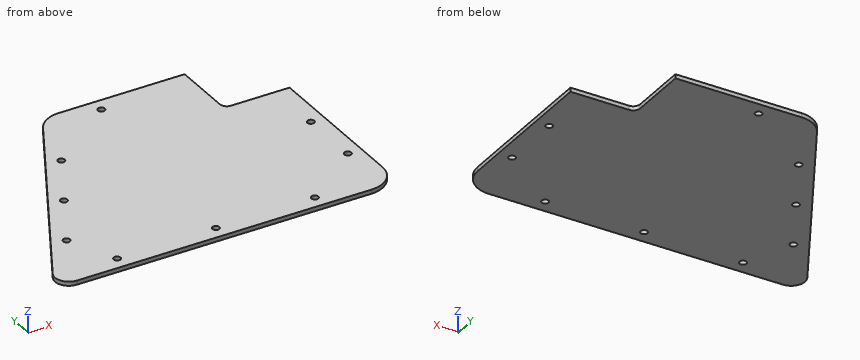
```python
from build123d import *

# Parameters (mm, degrees)
BOSS_EXTRUDE1_DEPTH = 3
CUT_EXTRUDE1_REACH  = 245.11
SKETCH2_R           = 2.5
CUT_EXTRUDE2_DEPTH  = 244.110466883


with BuildPart() as part:
    # Sketch1 → Boss-Extrude1 (new body)
    with BuildSketch(Plane.XY):
        with BuildLine():
            Line((-59.436088262, 179.5), (59.436088262, 179.5))
            ThreePointArc((59.436088262, 179.5), (73.578223886, 173.642135624), (79.436088262, 159.5))
            Line((79.436088262, 159.5), (79.436088262, 20))
            ThreePointArc((79.436088262, 20), (73.578223886, 5.857864376), (59.436088262, 0))
            Line((59.436088262, 0), (-153.931232863, 0))
            ThreePointArc((-153.931232863, 0), (-162.549941964, 4.928722701), (-162.672805625, 14.856429312))
            Line((-162.672805625, 14.856429312), (-76.919233785, 169.212858624))
            ThreePointArc((-76.919233785, 169.212858624), (-69.57864286, 176.737418201), (-59.436088262, 179.5))
        make_face()
    extrude(amount=BOSS_EXTRUDE1_DEPTH)

    # Sketch2 → Cut-Extrude1 (cut, up to next)
    with BuildSketch(Plane.XY.offset(3), mode=Mode.PRIVATE) as cut_extrude1_sk1:
        with Locations((-34.436088262, 169.5)):
            Circle(SKETCH2_R)
    cut_extrude1_tool1 = extrude(cut_extrude1_sk1.sketch, amount=-CUT_EXTRUDE1_REACH, mode=Mode.PRIVATE) & part.part
    # Sketch2 → Cut-Extrude1 (cut, up to next)
    with BuildSketch(Plane.XY.offset(3), mode=Mode.PRIVATE) as cut_extrude1_sk2:
        with Locations((34.433911738, 169.5)):
            Circle(SKETCH2_R)
    cut_extrude1_tool2 = extrude(cut_extrude1_sk2.sketch, amount=-CUT_EXTRUDE1_REACH, mode=Mode.PRIVATE) & part.part
    # Sketch2 → Cut-Extrude1 (cut, up to next)
    with BuildSketch(Plane.XY.offset(3), mode=Mode.PRIVATE) as cut_extrude1_sk3:
        with Locations((69.436088262, 134.5)):
            Circle(SKETCH2_R)
    cut_extrude1_tool3 = extrude(cut_extrude1_sk3.sketch, amount=-CUT_EXTRUDE1_REACH, mode=Mode.PRIVATE) & part.part
    # Sketch2 → Cut-Extrude1 (cut, up to next)
    with BuildSketch(Plane.XY.offset(3), mode=Mode.PRIVATE) as cut_extrude1_sk4:
        with Locations((69.436088262, 89.75)):
            Circle(SKETCH2_R)
    cut_extrude1_tool4 = extrude(cut_extrude1_sk4.sketch, amount=-CUT_EXTRUDE1_REACH, mode=Mode.PRIVATE) & part.part
    # Sketch2 → Cut-Extrude1 (cut, up to next)
    with BuildSketch(Plane.XY.offset(3), mode=Mode.PRIVATE) as cut_extrude1_sk5:
        with Locations((69.436088262, 45)):
            Circle(SKETCH2_R)
    cut_extrude1_tool5 = extrude(cut_extrude1_sk5.sketch, amount=-CUT_EXTRUDE1_REACH, mode=Mode.PRIVATE) & part.part
    # Sketch2 → Cut-Extrude1 (cut, up to next)
    with BuildSketch(Plane.XY.offset(3), mode=Mode.PRIVATE) as cut_extrude1_sk6:
        with Locations((24.436088262, 10)):
            Circle(SKETCH2_R)
    cut_extrude1_tool6 = extrude(cut_extrude1_sk6.sketch, amount=-CUT_EXTRUDE1_REACH, mode=Mode.PRIVATE) & part.part
    # Sketch2 → Cut-Extrude1 (cut, up to next)
    with BuildSketch(Plane.XY.offset(3), mode=Mode.PRIVATE) as cut_extrude1_sk7:
        with Locations((-47.243911738, 10)):
            Circle(SKETCH2_R)
    cut_extrude1_tool7 = extrude(cut_extrude1_sk7.sketch, amount=-CUT_EXTRUDE1_REACH, mode=Mode.PRIVATE) & part.part
    # Sketch2 → Cut-Extrude1 (cut, up to next)
    with BuildSketch(Plane.XY.offset(3), mode=Mode.PRIVATE) as cut_extrude1_sk8:
        with Locations((-118.923911738, 10)):
            Circle(SKETCH2_R)
    cut_extrude1_tool8 = extrude(cut_extrude1_sk8.sketch, amount=-CUT_EXTRUDE1_REACH, mode=Mode.PRIVATE) & part.part
    # Sketch2 → Cut-Extrude1 (cut, up to next)
    with BuildSketch(Plane.XY.offset(3), mode=Mode.PRIVATE) as cut_extrude1_sk9:
        with Locations((-134.505515616, 44.966291045)):
            Circle(SKETCH2_R)
    cut_extrude1_tool9 = extrude(cut_extrude1_sk9.sketch, amount=-CUT_EXTRUDE1_REACH, mode=Mode.PRIVATE) & part.part
    # Sketch2 → Cut-Extrude1 (cut, up to next)
    with BuildSketch(Plane.XY.offset(3), mode=Mode.PRIVATE) as cut_extrude1_sk10:
        with Locations((-87.602121323, 129.392400773)):
            Circle(SKETCH2_R)
    cut_extrude1_tool10 = extrude(cut_extrude1_sk10.sketch, amount=-CUT_EXTRUDE1_REACH, mode=Mode.PRIVATE) & part.part
    # Sketch2 → Cut-Extrude1 (cut, up to next)
    with BuildSketch(Plane.XY.offset(3), mode=Mode.PRIVATE) as cut_extrude1_sk11:
        with Locations((-111.05381847, 87.179345909)):
            Circle(SKETCH2_R)
    cut_extrude1_tool11 = extrude(cut_extrude1_sk11.sketch, amount=-CUT_EXTRUDE1_REACH, mode=Mode.PRIVATE) & part.part
    add(cut_extrude1_tool1.solids().sort_by_distance((-34.436088, 169.5, 3))[0], mode=Mode.SUBTRACT)
    add(cut_extrude1_tool2.solids().sort_by_distance((34.433912, 169.5, 3))[0], mode=Mode.SUBTRACT)
    add(cut_extrude1_tool3.solids().sort_by_distance((69.436088, 134.5, 3))[0], mode=Mode.SUBTRACT)
    add(cut_extrude1_tool4.solids().sort_by_distance((69.436088, 89.75, 3))[0], mode=Mode.SUBTRACT)
    add(cut_extrude1_tool5.solids().sort_by_distance((69.436088, 45, 3))[0], mode=Mode.SUBTRACT)
    add(cut_extrude1_tool6.solids().sort_by_distance((24.436088, 10, 3))[0], mode=Mode.SUBTRACT)
    add(cut_extrude1_tool7.solids().sort_by_distance((-47.243912, 10, 3))[0], mode=Mode.SUBTRACT)
    add(cut_extrude1_tool8.solids().sort_by_distance((-118.923912, 10, 3))[0], mode=Mode.SUBTRACT)
    add(cut_extrude1_tool9.solids().sort_by_distance((-134.505516, 44.966291, 3))[0], mode=Mode.SUBTRACT)
    add(cut_extrude1_tool10.solids().sort_by_distance((-87.602121, 129.392401, 3))[0], mode=Mode.SUBTRACT)
    add(cut_extrude1_tool11.solids().sort_by_distance((-111.053818, 87.179346, 3))[0], mode=Mode.SUBTRACT)

    # Sketch3 → Cut-Extrude2 (cut, through all)
    with BuildSketch(Plane.XY.offset(3)):
        with BuildLine():
            Line((31.933911738, 179.5), (31.933911738, 137))
            ThreePointArc((31.933911738, 137), (33.398377832, 133.464466094), (36.933911738, 132))
            Line((36.933911738, 132), (79.436088262, 132))
            Line((79.436088262, 132), (79.436088262, 159.5))
            ThreePointArc((79.436088262, 159.5), (73.578223886, 173.642135624), (59.436088262, 179.5))
            Line((59.436088262, 179.5), (31.933911738, 179.5))
        make_face()
    extrude(amount=-CUT_EXTRUDE2_DEPTH, mode=Mode.SUBTRACT)


solid = part.part
```
Design review of the part built by this model. Coordinates are the model's own, in mm. Round coordinates to 2 decimals unless told otherwise and drop trailing zeros. Order: outer loops, then holes, each group sorted by start corner. A loop starts at its lowest first (then second) coordinate and runs counter-clockwise, first axis right, second up. Notation, with made-up numbers: (25.5, 80) - (72.5, 80) arc R30 ccw to (72.5, 110) - close; hole circle Ø7 at (-26, 34.25). An arc over 180 degrees is marked (long way). Return JSON: item names as keys, results as strings.
Q1. For pin 1 Ø4.5 at (x, y) = (-118.92, 10) entering from -Z, flat-tipped, find the tip position at first contact; note if it passes through.
Computed values:
{"pin 1": "passes through"}
Q2. Consider section A-A on z = 1. Give the number of separate pieces and of enclosed holes in the cut face, plus the area to 3 significant figures.
Computed values:
{"separate pieces": "1", "enclosed holes": "9", "area": "33,400 mm2"}
Q3. Consider section D-D on y = 107. Write out the cut boundary in (x, z), plus the area to 3 significant figures.
Computed values:
{"outline": "(-111.48, 0) - (79.44, 0) - (79.44, 3) - (-111.48, 3) - close", "area": "573 mm2"}
Q4. Consider section B-B on y = 10. Write out the cut boundary in (x, z), plus the area to 3 significant figures.
Computed values:
{"outline": "(-163.93, 0) - (-121.42, 0) - (-121.42, 3) - (-163.93, 3) - close; (-116.42, 0) - (-49.74, 0) - (-49.74, 3) - (-116.42, 3) - close; (-44.74, 0) - (21.94, 0) - (21.94, 3) - (-44.74, 3) - close; (26.94, 0) - (76.76, 0) - (76.76, 3) - (26.94, 3) - close", "area": "677 mm2"}
Q5. Consider section C-C on x = 53. Write out the cut boundary in (y, z).
Computed values:
{"outline": "(0, 0) - (132, 0) - (132, 3) - (0, 3) - close"}
Q6. Wall thickness on L1, parallel to Y at x = -136, z = 2.95; L2, parallel to Y at x = 36.5, z = 2.95; L3, parallel to X at y = 113, z = 2.25: over which ranges is each line inside the solid? List them lowest first. Write a range as [from, to].
Computed values:
{"L1": "y = [0, 42.96], [46.97, 62.87]", "L2": "y = [0, 132.02]", "L3": "x = [-108.15, 79.44]"}
